Work out the finished part from the listing and answer in its coordinate system (mm). Round coordinates to 2 decimals unless told otherwise and drop trailing zeros. One line per item, written item: value.
```python
from build123d import *

# Parameters (mm, degrees)
SKETCH1_R           = 2.1
BOSS_EXTRUDE1_DEPTH = 503


with BuildPart() as part:
    # Sketch1 → Boss-Extrude1 (new body)
    with BuildSketch(Plane.XY):
        with BuildLine():
            Line((0, 1), (0, 5.36))
            Line((0, 5.36), (1.8, 7.16))
            Line((1.8, 7.16), (1.8, 4.500660172))
            Line((1.8, 4.500660172), (3.44, 4.500660172))
            Line((3.44, 4.500660172), (6.099339828, 7.16))
            Line((6.099339828, 7.16), (6.099339828, 12.84))
            Line((6.099339828, 12.84), (3.44, 15.499339828))
            Line((3.44, 15.499339828), (1.8, 15.499339828))
            Line((1.8, 15.499339828), (1.8, 12.84))
            Line((1.8, 12.84), (0, 14.64))
            Line((0, 14.64), (0, 19))
            ThreePointArc((0, 19), (0.292893219, 19.707106781), (1, 20))
            Line((1, 20), (5.36, 20))
            Line((5.36, 20), (7.16, 18.2))
            Line((7.16, 18.2), (4.500660172, 18.2))
            Line((4.500660172, 18.2), (4.500660172, 16.56))
            Line((4.500660172, 16.56), (7.16, 13.900660172))
            Line((7.16, 13.900660172), (12.84, 13.900660172))
            Line((12.84, 13.900660172), (15.464579042, 16.525239214))
            Line((15.464579042, 16.525239214), (15.464579042, 18.165239214))
            Line((15.464579042, 18.165239214), (12.84, 18.2))
            Line((12.84, 18.2), (14.64, 20))
            Line((14.64, 20), (19, 20))
            ThreePointArc((19, 20), (19.707106781, 19.707106781), (20, 19))
            Line((20, 19), (20, 14.674581351))
            Line((20, 14.674581351), (18.155899385, 12.84))
            Line((18.155899385, 12.84), (18.155899385, 15.455239214))
            Line((18.155899385, 15.455239214), (16.515899385, 15.455239214))
            Line((16.515899385, 15.455239214), (13.900660172, 12.84))
            Line((13.900660172, 12.84), (13.900660172, 7.16))
            Line((13.900660172, 7.16), (16.56, 4.500660172))
            Line((16.56, 4.500660172), (18.2, 4.500660172))
            Line((18.2, 4.500660172), (18.2, 7.16))
            Line((18.2, 7.16), (20, 5.36))
            Line((20, 5.36), (20, 1))
            ThreePointArc((20, 1), (19.707106781, 0.292893219), (19, 0))
            Line((19, 0), (14.64, 0))
            Line((14.64, 0), (12.84, 1.8))
            Line((12.84, 1.8), (15.499339828, 1.8))
            Line((15.499339828, 1.8), (15.499339828, 3.44))
            Line((15.499339828, 3.44), (12.84, 6.099339828))
            Line((12.84, 6.099339828), (7.16, 6.099339828))
            Line((7.16, 6.099339828), (4.500660172, 3.44))
            Line((4.500660172, 3.44), (4.500660172, 1.8))
            Line((4.500660172, 1.8), (7.16, 1.8))
            Line((7.16, 1.8), (5.36, 0))
            Line((5.36, 0), (1, 0))
            ThreePointArc((1, 0), (0.292893219, 0.292893219), (0, 1))
        make_face()
        with Locations((10.02040103, 9.97959897)):
            Circle(SKETCH1_R, mode=Mode.SUBTRACT)
        Polygon((16.534579042, 18.2), (16.534579042, 17.576559557), (17.585899385, 16.525239214), (18.2, 16.525239214), (18.2, 18.2), align=None, mode=Mode.SUBTRACT)
        Polygon((18.2, 1.75919794), (18.2, 3.433958726), (17.585899385, 3.433958726), (16.534579042, 2.382638382), (16.534579042, 1.75919794), align=None, mode=Mode.SUBTRACT)
        Polygon((2.454902675, 16.525239214), (1.84080206, 16.525239214), (1.84080206, 18.2), (3.506223018, 18.2), (3.506223018, 17.576559557), align=None, mode=Mode.SUBTRACT)
        Polygon((3.506223018, 1.75919794), (1.84080206, 1.75919794), (1.84080206, 3.433958726), (2.454902675, 3.433958726), (3.506223018, 2.382638382), align=None, mode=Mode.SUBTRACT)
    extrude(amount=-BOSS_EXTRUDE1_DEPTH)


solid = part.part
```
1) Find section A-A (z = -192.5). Give the number of separate pieces and of enclosed holes in the cut face, then the cut area to 3 significant figures.
Check values:
separate pieces: 1
enclosed holes: 5
area: 162 mm2
2) Each of these flat-tipped pins is pushed along its axis until it touches: pin 1 (6 mm diameter, centred on x = 9.5, z = -243.5, fed in from +Y); pin 2 (2 mm diameter, centred on y = 6.5, z = -252, fed in from +X); pin 3 (5 mm diameter, centred on y = 9, z = -373.5, fed in from -X). Where does it stop, or does it pass through?
Check values:
pin 1: y = 18.86
pin 2: x = 19.86
pin 3: x = 1.14
3) Find the intervals of material crossed by probe 1 along Y at (x, z) = (2.25, -336); probe 2 along X at (y, z) = (2.25, -423); probe 3 along Y at (x, z) = (10, -327.5), in increasing order. Write a range as from..to.
Check values:
probe 1: 0..1.76, 3.43..4.5, 15.5..16.53, 18.2..20
probe 2: 0..1.84, 3.51..4.5, 15.5..16.53, 18.2..20
probe 3: 6.1..7.88, 12.08..13.9
